```python
from build123d import *

# Parameters (mm, degrees)
SKETCH1_R           = 2.4892
SKETCH1_R_2         = 3.175
BOSS_EXTRUDE2_DEPTH = 1.143
FILLET1_R           = 3.175
FILLET2_R           = 3.175
SKETCH2_OUTSIDE_W   = 197.508
SKETCH2_OUTSIDE_H   = 197.508
SKETCH2_OUTSIDE_W_2 = 152.4
SKETCH2_OUTSIDE_H_2 = 152.4
CUT_EXTRUDE1_DEPTH  = 2.54
FILLET3_R           = 2.54


with BuildPart() as part:
    # Sketch1 → Boss-Extrude2 (new, symmetric)
    with BuildSketch(Plane(origin=(0, 0, 0), x_dir=(1, 0, 0), z_dir=(0, 1, 0))):
        Polygon((0, 0), (0, 152.4), (-25.4, 152.4), (-152.4, 25.4), (-152.4, 0), align=None)
        with Locations(Location((-12.7, 12.7, 0), (0, 0, 270))):
            Circle(SKETCH1_R, mode=Mode.SUBTRACT)
        with Locations(Location((-38.1, 12.7, 0), (0, 0, 270))):
            Circle(SKETCH1_R, mode=Mode.SUBTRACT)
        with Locations(Location((-63.5, 12.7, 0), (0, 0, 270))):
            Circle(SKETCH1_R, mode=Mode.SUBTRACT)
        with Locations(Location((-88.9, 12.7, 0), (0, 0, 270))):
            Circle(SKETCH1_R, mode=Mode.SUBTRACT)
        with Locations(Location((-114.3, 12.7, 0), (0, 0, 270))):
            Circle(SKETCH1_R, mode=Mode.SUBTRACT)
        with Locations(Location((-12.7, 38.1, 0), (0, 0, 270))):
            Circle(SKETCH1_R, mode=Mode.SUBTRACT)
        with Locations(Location((-12.7, 63.5, 0), (0, 0, 270))):
            Circle(SKETCH1_R, mode=Mode.SUBTRACT)
        with Locations(Location((-12.7, 88.9, 0), (0, 0, 270))):
            Circle(SKETCH1_R, mode=Mode.SUBTRACT)
        with Locations(Location((-12.7, 114.3, 0), (0, 0, 270))):
            Circle(SKETCH1_R, mode=Mode.SUBTRACT)
        with Locations(Location((-139.7, 12.7, 0), (0, 0, 270))):
            Circle(SKETCH1_R, mode=Mode.SUBTRACT)
        with Locations(Location((-12.7, 139.7, 0), (0, 0, 270))):
            Circle(SKETCH1_R, mode=Mode.SUBTRACT)
        with Locations(Location((-101.6, 50.8, 0), (0, 0, 270))):
            Circle(SKETCH1_R_2, mode=Mode.SUBTRACT)
    extrude(amount=BOSS_EXTRUDE2_DEPTH, both=True)

    # Fillet1
    fillet1_edges = [part.edges().sort_by_distance(p)[0] for p in [
        (-152.4, 0, 0),
        (0, 0, 0),
    ]]
    fillet(fillet1_edges, radius=FILLET1_R)

    # Fillet2
    fillet2_edges = [part.edges().sort_by_distance(p)[0] for p in [
        (-152.4, 0, -25.4),
        (-25.4, 0, -152.4),
        (0, 0, -152.4),
    ]]
    fillet(fillet2_edges, radius=FILLET2_R)

    # Sketch2 outside → Cut-Extrude1 (cut)
    # profile 1 of 2: a face of its own
    with BuildSketch(Plane(origin=(0, 1.143, 0), x_dir=(1, 0, 0), z_dir=(0, 1, 0))):
        with Locations((-76.2, 76.2)):
            Rectangle(SKETCH2_OUTSIDE_W, SKETCH2_OUTSIDE_H)
        with Locations((-76.2, 76.2)):
            Rectangle(SKETCH2_OUTSIDE_W_2, SKETCH2_OUTSIDE_H_2, mode=Mode.SUBTRACT)
    # profile 2 of 2: a face of its own
    with BuildSketch(Plane(origin=(0, 1.143, 0), x_dir=(1, 0, 0), z_dir=(0, 1, 0))):
        Polygon((-38.1, 85.818463274), (-85.818463274, 38.1), (-38.1, 38.1), align=None)
    extrude(amount=-CUT_EXTRUDE1_DEPTH, mode=Mode.SUBTRACT)

    # Fillet3
    fillet3_edges = [part.edges().sort_by_distance(p)[0] for p in [
        (-38.1, 0, -85.818463274),
        (-38.1, 0, -38.1),
        (-85.818463274, 0, -38.1),
    ]]
    fillet(fillet3_edges, radius=FILLET3_R)


solid = part.part
```
Geometry: final body of the model. Coordinates: model frame, mm. A direction names the side the tool comes from. Coordinates: 2 decimals unless noted, no trailing zeros. Order: outer loops, then holes, each group sorted by start corner. A loop starts at its lowest first (then second) coordinate and runs counter-clockwise, first axis right, second up. Notation, with made-up numbers: (71, 16) -> (126, 16) arc R27 ccw to (126, 48) -> close; hole circle Ø3 at (-22, 40). An arc over 180 degrees is marked (long way). Write each question's results on one line, items separated by ' | '. Start each with the question number.
1) Cut plane A-A, the plane z = -12.7. Output: boundary loops of the cut face in (x, y).
2) Material intervals for line 1 along X through (y, z) = (0.3, -39.5); line 2 along X through (y, z) = (-0.35, -61.5); line 3 along X through (y, z) = (0.15, -88.9), sorted ascending.
3) First-contact query: pin 1 (4.5 mm diameter, centred on x = -12.7, z = -114.3, fed in from -Y); pin 2 (1.1 mm diameter, centred on y = 0, z = -69.5, fed in from -X); pin 3 (1.1 mm diameter, centred on x = -57.5, y = 0, fed in from -Z). Flat tips, straight axial feed; report the tip coordinate or a pass-through.
4) Set-up query: faces 1 (the flat face through (-77, -1.143, -60)), 2 (the flat face through (-61.69, 0.02, -62.23)). Return all of +Z, -Z, +X, -X, +Y, -Y with unobstructed straight access to the full face (end or side cutting, diameter ignored); none if empty.
5) Mould query, pull axis X, two halves, no side actions, for faces 3 (the cylindrical face through (-35.63, -0.02, -13.02)), 4 (the flat face through (-77, 1.143, -60)), 5 (the flat face through (-88, 0, -89.8)). Classes: released by +X, released by -X, zero draft, split by the parting line, or undercut.
6) Cut plane B-B, the plane z = -88.9. Output: boundary loops of the cut face in (x, y), and give its area (3 significant figures).
7) Cut plane D-D, the plane x = -101.6. Output: boundary loops of the cut face in (y, z) (3 decimals).
8) Cut plane C-C, the plane x = -12.7. Output: boundary loops of the cut face in (y, z).
Checks:
1) outline: (-152.4, -1.14) -> (-142.19, -1.14) -> (-142.19, 1.14) -> (-152.4, 1.14) -> close; (-137.21, -1.14) -> (-116.79, -1.14) -> (-116.79, 1.14) -> (-137.21, 1.14) -> close; (-111.81, -1.14) -> (-91.39, -1.14) -> (-91.39, 1.14) -> (-111.81, 1.14) -> close; (-86.41, -1.14) -> (-65.99, -1.14) -> (-65.99, 1.14) -> (-86.41, 1.14) -> close; (-61.01, -1.14) -> (-40.59, -1.14) -> (-40.59, 1.14) -> (-61.01, 1.14) -> close; (-35.61, -1.14) -> (-15.19, -1.14) -> (-15.19, 1.14) -> (-35.61, 1.14) -> close; (-10.21, -1.14) -> (0, -1.14) -> (0, 1.14) -> (-10.21, 1.14) -> close
2) line 1: -138.3 to -81.96, -38.37 to -14.76, -10.64 to 0 | line 2: -116.3 to -62.42, -38.1 to -14.18, -11.22 to 0 | line 3: -88.9 to -15.19, -10.21 to 0
3) pin 1: through | pin 2: x = -108.85 | pin 3: z = -120.85
4) face 1: +Z, -Z, +X, -X, -Y | face 2: +Y, -Y
5) face 3: undercut | face 4: zero draft | face 5: released by -X
6) outline: (-88.9, -1.14) -> (-15.19, -1.14) -> (-15.19, 1.14) -> (-88.9, 1.14) -> close; (-10.21, -1.14) -> (0, -1.14) -> (0, 1.14) -> (-10.21, 1.14) -> close | area: 192 mm^2
7) outline: (-1.143, -76.2) -> (1.143, -76.2) -> (1.143, -53.975) -> (-1.143, -53.975) -> close; (-1.143, -47.625) -> (1.143, -47.625) -> (1.143, 0) -> (-1.143, 0) -> close
8) outline: (-1.14, -152.4) -> (1.14, -152.4) -> (1.14, -142.19) -> (-1.14, -142.19) -> close; (-1.14, -137.21) -> (1.14, -137.21) -> (1.14, -116.79) -> (-1.14, -116.79) -> close; (-1.14, -111.81) -> (1.14, -111.81) -> (1.14, -91.39) -> (-1.14, -91.39) -> close; (-1.14, -86.41) -> (1.14, -86.41) -> (1.14, -65.99) -> (-1.14, -65.99) -> close; (-1.14, -61.01) -> (1.14, -61.01) -> (1.14, -40.59) -> (-1.14, -40.59) -> close; (-1.14, -35.61) -> (1.14, -35.61) -> (1.14, -15.19) -> (-1.14, -15.19) -> close; (-1.14, -10.21) -> (1.14, -10.21) -> (1.14, 0) -> (-1.14, 0) -> close
